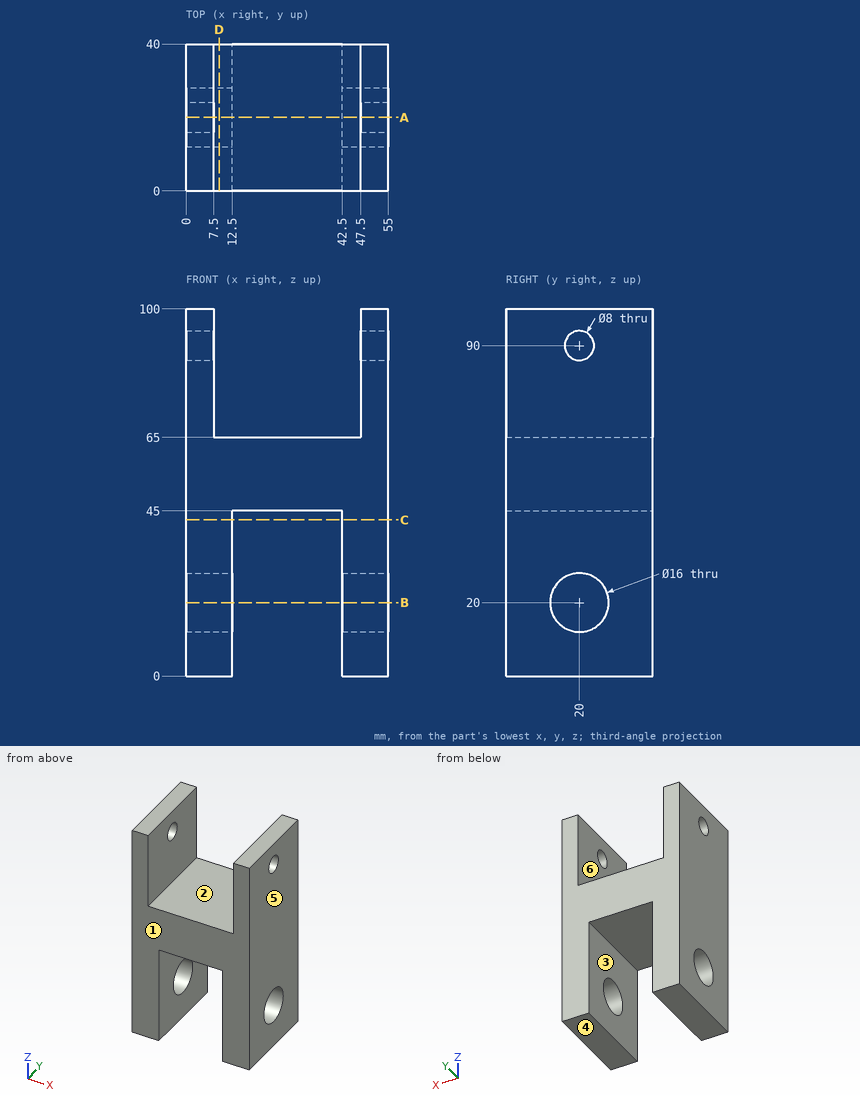
Answer from the drawing. Dimensions are ordinates in mm from the lowest x, y and z of the part. A direction names the side the tool comes from. Round coordinates to 2 decimals unless told otherwise and drop trailing zeros. Loops run counter-clockwise (first coordinate to the right, second up) from the corner with the lowest first, then second, coordinate; pieces in that order, holes last.
Q1. Determine the mould class of the marked faces 4, 5 and 6 for opening direction X: released by +X, released by -X, zero draft, split by the parting line, or undercut.
Q2. Section B-B on z = 20 is taken. Write down the section's boundary in (x, y).
Q3. Consider probe 1 along Z at (x, y) = (7, 20); probe 2 along X at (y, z) = (38.5, 13); probe 3 along X at (y, z) = (13.5, 81). Determine where each line is inside the solid, lowest interval first.
Q4. Which of the six approach directions +Z, -Z, +X, -X, +Y, -Y give full straight-line access (tool end or side, diameter ignored) to the marked faces 1, 2 and 3?
Q5. This flat-tipped pin is pushed along its axis until it touches: pin 1 (18.5 mm diameter, centred on y = 20, z = 20, fed in from -X). Where does it stop, or does it pass through?
Q6. Section D-D on x = 9 is taken. Write down the section's boundary in (y, z), and give its area (3 significant figures).
Q7. Section A-A on y = 20 is taken. Write down the section's boundary in (x, z), and give its area (3 significant figures).
Q8. Section C-C on z = 42.5 is taken. Write down the section's boundary in (x, y).
Output:
1. face 4: zero draft
1. face 5: released by +X
1. face 6: undercut
2. outline: (0, 0) - (12.5, 0) - (12.5, 12) - (0, 12) - close; (0, 28) - (12.5, 28) - (12.5, 40) - (0, 40) - close; (42.5, 0) - (55, 0) - (55, 12) - (42.5, 12) - close; (42.5, 28) - (55, 28) - (55, 40) - (42.5, 40) - close
3. probe 1: z = 0 to 12, 28 to 86, 94 to 100
3. probe 2: x = 0 to 12.5, 42.5 to 55
3. probe 3: x = 0 to 7.5, 47.5 to 55
4. face 1: +Z, -Z, +X, -X, -Y
4. face 2: +Z, +Y, -Y
4. face 3: -Z, +Y, -Y
5. pin 1: stops at x = 0
6. outline: (0, 0) - (40, 0) - (40, 65) - (0, 65) - close; hole circle Ø16 at (20, 20)
6. area: 2,400 mm2
7. outline: (0, 0) - (12.5, 0) - (12.5, 12) - (0, 12) - close; (0, 28) - (12.5, 28) - (12.5, 45) - (42.5, 45) - (42.5, 28) - (55, 28) - (55, 86) - (47.5, 86) - (47.5, 65) - (7.5, 65) - (7.5, 86) - (0, 86) - close; (0, 94) - (7.5, 94) - (7.5, 100) - (0, 100) - close; (42.5, 0) - (55, 0) - (55, 12) - (42.5, 12) - close; (47.5, 94) - (55, 94) - (55, 100) - (47.5, 100) - close
7. area: 2,230 mm2
8. outline: (0, 0) - (12.5, 0) - (12.5, 40) - (0, 40) - close; (42.5, 0) - (55, 0) - (55, 40) - (42.5, 40) - close
